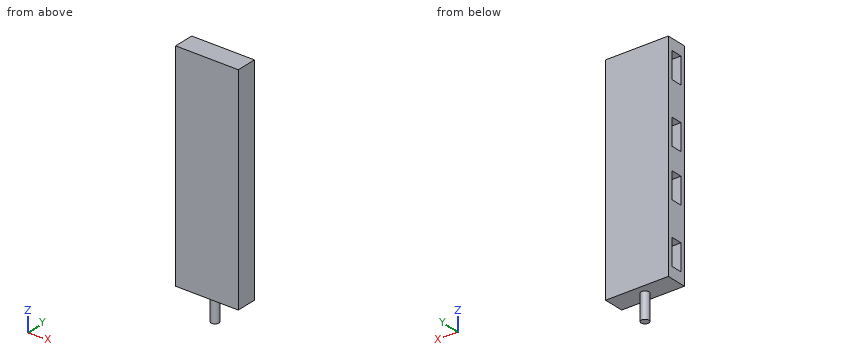
Autodesk Inventor part; units mm, degrees
ref_plane "YZ Plane" through (0, 0, 0) normal (1, 0, 0) x (0, 1, 0)
ref_plane "XZ Plane" through (0, 0, 0) normal (0, 1, 0) x (-1, 0, 0)
ref_plane "XY Plane" through (0, 0, 0) normal (0, 0, 1) x (1, 0, 0)
sketch "Sketch1" plane through (0, 0, 0) normal (0, 1, 0) x (-1, 0, 0)
  line L0 (15.621, 53.721) -> (-15.621, 53.721)
  line L1 (-15.621, 53.721) -> (-15.621, -53.721)
  line L2 (-15.621, -53.721) -> (15.621, -53.721)
  line L3 (15.621, -53.721) -> (15.621, 53.721)
  line L4 (15.621, 53.721) -> (-15.621, -53.721) construction
  line L5 (-15.621, 53.721) -> (15.621, -53.721) construction
  point P0 (0, 0)
  dimension "d0" = 107.442
  dimension "d1" = 31.242
extrude "Extrusion1" add sketch "Sketch1" along normal blind 10.16
sketch "Sketch2" plane through (-15.621, 0, -53.721) normal (-1, 0, 0) x (0, 0, 1)
  line L0 (0, 0) -> (0, 10.16)
  line L1 (0, 5.08) -> (107.442, 5.08) construction
  line L2 (107.442, 0) -> (107.442, 10.16)
  line L3 (107.442, 10.16) -> (0, 10.16)
  line L4 (53.721, 10.16) -> (53.721, 0) construction
  line L5 (107.442, 0) -> (0, 0)
  line L6 (35.2574, 2.1925) -> (48.2344, 2.1925)
  line L7 (48.2344, 2.1925) -> (48.2344, 7.9675)
  line L8 (48.2344, 7.9675) -> (35.2574, 7.9675)
  line L9 (35.2574, 7.9675) -> (35.2574, 2.1925)
  line L10 (35.2574, 2.1925) -> (48.2344, 7.9675) construction
  line L11 (48.2344, 2.1925) -> (35.2574, 7.9675) construction
  line L12 (0, 10.16) -> (53.721, 10.16)
  line L13 (26.8605, 10.16) -> (26.8605, 0) construction
  line L14 (18.4636, 2.1925) -> (5.4866, 2.1925)
  line L15 (5.4866, 2.1925) -> (5.4866, 7.9675)
  line L16 (5.4866, 7.9675) -> (18.4636, 7.9675)
  line L17 (18.4636, 7.9675) -> (18.4636, 2.1925)
  line L18 (18.4636, 2.1925) -> (5.4866, 7.9675) construction
  line L19 (5.4866, 2.1925) -> (18.4636, 7.9675) construction
  line L20 (107.442, 5.08) -> (0, 5.08) construction
  line L21 (72.1846, 2.1925) -> (59.2076, 2.1925)
  line L22 (59.2076, 2.1925) -> (59.2076, 7.9675)
  line L23 (59.2076, 7.9675) -> (72.1846, 7.9675)
  line L24 (72.1846, 7.9675) -> (72.1846, 2.1925)
  line L25 (72.1846, 2.1925) -> (59.2076, 7.9675) construction
  line L26 (59.2076, 2.1925) -> (72.1846, 7.9675) construction
  line L27 (80.5815, 10.16) -> (80.5815, 0) construction
  line L28 (88.9784, 2.1925) -> (101.9554, 2.1925)
  line L29 (101.9554, 2.1925) -> (101.9554, 7.9675)
  line L30 (101.9554, 7.9675) -> (88.9784, 7.9675)
  line L31 (88.9784, 7.9675) -> (88.9784, 2.1925)
  line L32 (88.9784, 2.1925) -> (101.9554, 7.9675) construction
  line L33 (101.9554, 2.1925) -> (88.9784, 7.9675) construction
  point P0 (41.7459, 5.08)
  point P1 (11.9751, 5.08)
  point P2 (65.6961, 5.08)
  point P3 (95.4669, 5.08)
extrude "Extrusion2" cut sketch "Sketch2" against normal blind 10.16 contours L9 L8 L7 L6 | L14 L15 L16 L17 | L21 L22 L23 L24 | L31 L30 L29 L28
sketch "Sketch3" plane through (15.621, 0, -53.721) normal (0, 0, -1) x (-1, 0, 0)
  line L0 (0, 10.16) -> (31.242, 10.16)
  line L1 (15.621, 10.16) -> (15.621, 0) construction
  circle A0 centre (15.621, 5.08) radius 1.905
  dimension "d6" = 3.81
extrude "Extrusion3" add sketch "Sketch3" along normal blind 12.7
properties part number "anker_4-port_usb3.0_splitter"
Verification items for the finished model (mm, model axes). Coordinates: 2 decimals unless noted, no trailing zeros. Write each loop counter-clockwise with the first axis right and the second up, starting at its lowest first coordinate (ties: lowest second). Pieces come first, ordered by that corner, then holes. Notation, with made-up numbers: M -12,27.25 L -5,27.25 A26 ccw -5,51.25 Z; hole C 45,76.5 d2. An arc over 180 degrees is marked long. Use CSV: the item, a comma, the result in double quotes.
Q1. Thickness scan on line 1 along Z through (x, y) = (-9.5, 5.5); line 2 along Z through (x, y) = (9.5, 5.5); line 3 along X through (y, z) = (2.5, -9). Record the ranges inside material, lowest first. Write a range as [from, to].
Computed values:
line 1,"[-53.72, -48.23], [-35.26, -18.46], [-5.49, 5.49], [18.46, 35.26], [48.23, 53.72]"
line 2,"[-53.72, 53.72]"
line 3,"[-5.46, 15.62]"
Q2. Section check B-B, the plane x = -12. Enter the section's corners in (y, z).
Computed values:
outline,"M 0,-53.72 L 10.16,-53.72 L 10.16,53.72 L 0,53.72 Z; hole M 2.19,-48.23 L 7.97,-48.23 L 7.97,-35.26 L 2.19,-35.26 Z; hole M 2.19,-18.46 L 7.97,-18.46 L 7.97,-5.49 L 2.19,-5.49 Z; hole M 2.19,5.49 L 7.97,5.49 L 7.97,18.46 L 2.19,18.46 Z; hole M 2.19,35.26 L 7.97,35.26 L 7.97,48.23 L 2.19,48.23 Z"
Q3. Section check C-C, the plane z = 15.5. Enter the section's corners in (x, y), and give its area (3 significant figures).
Computed values:
outline,"M -15.62,0 L 15.62,0 L 15.62,10.16 L -15.62,10.16 L -15.62,7.97 L -5.46,7.97 L -5.46,2.19 L -15.62,2.19 Z"
area,"259 mm²"
Q4. Section check D-D, the plane y = 5.08. Enter the section's corners in (x, z) (3 decimals).
Computed values:
outline,"M -15.621,-53.721 L -1.905,-53.721 L -1.905,-66.421 L 1.905,-66.421 L 1.905,-53.721 L 15.621,-53.721 L 15.621,53.721 L -15.621,53.721 L -15.621,48.234 L -5.461,48.234 L -5.461,35.257 L -15.621,35.257 L -15.621,18.464 L -5.461,18.464 L -5.461,5.487 L -15.621,5.487 L -15.621,-5.487 L -5.461,-5.487 L -5.461,-18.464 L -15.621,-18.464 L -15.621,-35.257 L -5.461,-35.257 L -5.461,-48.234 L -15.621,-48.234 Z"
Q5. Go/stop test with flat-tipped pins: P1, Ø3, axis at x = -10, z = -40.5, coming from the -Y side; P2, Ø1.7, axis at x = -13, y = 5.5, coming from the -Z side; P3, Ø1.7, axis at y = 3.5, z = -41, coming from the -X side. Record where each tip stops, or that it passes through.
Computed values:
P1,"y = 0"
P2,"z = -53.72"
P3,"x = -5.46"
Q6. Section check A-A, the plane x = 0. Enter the section's corners in (y, z) (3 decimals).
Computed values:
outline,"M 0,-53.721 L 3.175,-53.721 L 3.175,-66.421 L 6.985,-66.421 L 6.985,-53.721 L 10.16,-53.721 L 10.16,53.721 L 0,53.721 Z"
